Check sheet for the drawn part. Datum: minimum x, y, z corner. Units: mm. Give positions to 0.01 mm unless a question says otherwise; leave off trailing zeros. Order: outer loops, then holes, each group sorted by start corner. A loop starts at its lowest first (then second) coordinate and runs counter-clockwise, first axis right, second up. Notation, with made-up numbers: (17.25, 68) -> (73.25, 68) arc R32 cw to (73.25, 101) -> close; hole circle Ø5 at (65, -5.5). An arc over 180 degrees is marked (long way). Answer in a Markdown table with one row per item. Add a question column.
(1) Cross-section at B-B (x = 1.05). State how many separate pieces and enclosed holes the cut face has, then the cut area to 3 significant figures.
(2) Thickness scan on L1, parallel to Y at x = 1.6, z = 28.05 (1 decimal); L2, parallel to Z at x = 2.85, y = 28.5; L3, parallel to Y at x = 2.2, z = 25.5 (1 decimal). Record the ranges inside material, lowest first. Write a range as [from, to].
(3) Go/stop test with flat-tipped pins: pin 1 (1.5 mm diameter, centred on x = 3, y = 50, fed in from +Z); pin 2 (8.5 mm diameter, centred on y = 108.825, z = 48.15, fed in from +X); pin 3 (1.5 mm diameter, centred on x = 1, y = 68, fed in from -Z). Record where each tip stops, or that it passes through.
(4) Cross-section at D-D (z = 12.7). Record the cut outline in (x, y) (1 decimal).
(5) Cross-section at C-C (y = 103.5). Record the cut outline in (x, z).
(6) Cross-section at A-A (z = 47.5). Record the cut outline in (x, y) (1 decimal).
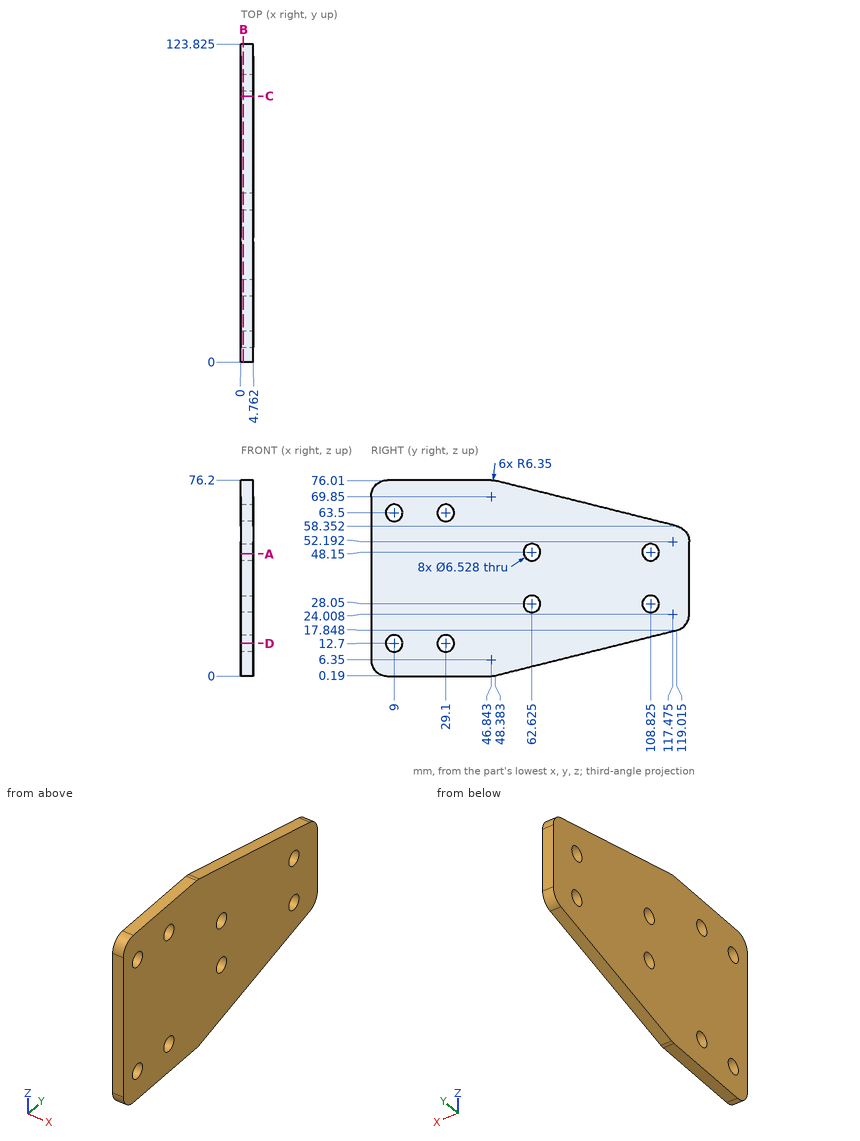
Answer below:
| question | item | result |
|---|---|---|
| 1 | separate pieces | 1 |
| 1 | enclosed holes | 8 |
| 1 | area | 7,690 mm² |
| 2 | L1 | y = [0, 59.4], [65.9, 105.6], [112.1, 123.8] |
| 2 | L2 | z = [0, 9.49], [15.91, 60.29], [66.71, 76.2] |
| 2 | L3 | y = [0, 60.6], [64.7, 106.8], [110.9, 123.8] |
| 3 | pin 1 | stops at z = 75.79 |
| 3 | pin 2 | stops at x = 4.76 |
| 3 | pin 3 | stops at z = 4.91 |
| 4 | outline | (0, 0) -> (4.8, 0) -> (4.8, 5.7) -> (0, 5.7) -> close; (0, 12.3) -> (4.8, 12.3) -> (4.8, 25.8) -> (0, 25.8) -> close; (0, 32.4) -> (4.8, 32.4) -> (4.8, 98.4) -> (0, 98.4) -> close |
| 5 | outline | (0, 13.97) -> (4.76, 13.97) -> (4.76, 62.23) -> (0, 62.23) -> close |
| 6 | outline | (0, 0) -> (4.8, 0) -> (4.8, 59.4) -> (0, 59.4) -> close; (0, 65.8) -> (4.8, 65.8) -> (4.8, 105.6) -> (0, 105.6) -> close; (0, 112) -> (4.8, 112) -> (4.8, 123.8) -> (0, 123.8) -> close |
